Geometry check sheet. Reference: drawing and pictorial views, mm from the part's lowest x, y, z. Give positions to 0.01 mm unless a question says otherwise; leave off trailing zeros. Order: outer loops, then holes, each group sorted by start corner. A loop starts at its lowest first (then second) coordinate and runs counter-clockwise, first axis right, second up.
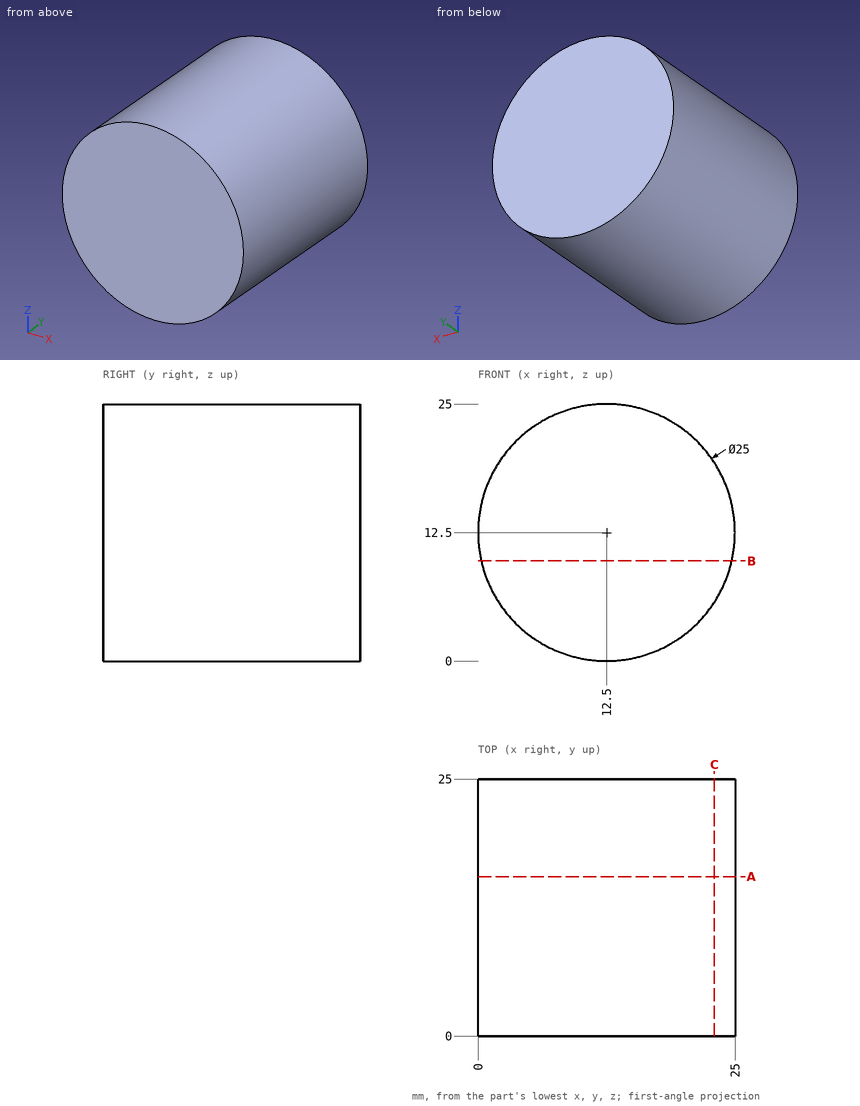
(1) Cross-section at B-B on z = 9.75. Enter the section's corners in (x, y).
Response values:
outline: (0.31, 0) - (24.69, 0) - (24.69, 25) - (0.31, 25) - close
(2) Gauge pin test, flat ends, axial feed: pin 1 Ø5 at (x, y) = (16, 4.5) entering from -Z; pin 2 Ø8 at (x, y) = (20.5, 5.5) entering from +Z; pin 3 Ø6 at (y, z) = (4, 15) entering from -X; pin 4 Ø12 at (y, z) = (10, 19) entering from +X. Record the tip position at first contact, or that the pin passes through.
Response values:
pin 1: stops at z = 0.04
pin 2: stops at z = 24.34
pin 3: stops at x = 0
pin 4: stops at x = 24.99
(3) Cross-section at A-A on y = 15.5. Enter the section's corners in (x, z).
Response values:
outline: circle Ø25 at (12.5, 12.5)
(4) Cross-section at C-C on x = 23. Enter the section's corners in (y, z), then the cut area to 3 significant figures.
Response values:
outline: (0, 5.72) - (25, 5.72) - (25, 19.28) - (0, 19.28) - close
area: 339 mm2
(5) Material ranges on L1, parallel to X at y = 8.25, z = 19.5; L2, parallel to X at y = 7.75, z = 16; L3, parallel to Z at x = 13.75, y = 12.5, recorded low to high.
Response values:
L1: x = 2.14 to 22.86
L2: x = 0.5 to 24.5
L3: z = 0.06 to 24.94
